Autodesk Inventor part; units mm, degrees
ref_plane "YZ Plane" through (0, 0, 0) normal (1, 0, 0) x (0, 1, 0)
ref_plane "XZ Plane" through (0, 0, 0) normal (0, 1, 0) x (-1, 0, 0)
ref_plane "XY Plane" through (0, 0, 0) normal (0, 0, 1) x (1, 0, 0)
sketch "Skizze1" plane through (0, 0, 0) normal (0, 1, 0) x (-1, 0, 0)
  line L0 (0, 0) -> (20, 0)
  line L1 (20, 0) -> (20, 40)
  line L2 (20, 40) -> (0, 40)
  line L3 (0, 40) -> (0, 0)
  circle A0 centre (10, 33) radius 2.55
  circle A1 centre (10, 7) radius 2.55
  dimension "d0" = 20
  dimension "d1" = 40
  dimension "d2" = 5.1
  dimension "d3" = 5.1
  dimension "d4" = 7
  dimension "d5" = 7
  dimension "d6" = 10
  dimension "d7" = 10
extrude "Extrusion1" add sketch "Skizze1" along normal blind 5
fillet "Rundung1" radius 2 4 edges at (-20, 2.5, 40) (-20, 2.5, 0) (0, 2.5, 0) (0, 2.5, 40)
sketch "Skizze2" plane through (0, 5, 0) normal (0, 1, 0) x (1, 0, 0)
  line L0 (-20, -2) -> (-20, -38)
  line L1 (-20, -25) -> (0, -25)
  line L2 (0, -25) -> (0, -15)
  line L3 (0, -15) -> (-20, -15)
  line L4 (-20, -15) -> (-20, -25)
  line L5 (-2, 0) -> (-18, 0)
  line L6 (-18, -40) -> (-2, -40)
  point P0 (0, 0)
  dimension "d11" = 10
  dimension "d12" = 20
  dimension "d13" = 15
  dimension "d14" = 15
sketch "Skizze5" plane through (0, 0, 0) normal (1, 0, 0) x (0, 1, 0)
  line L0 (55, 21) -> (55, 19)
  line L1 (5, 0) -> (0, 0)
  line L2 (5, 2) -> (5, 38)
  line L3 (5, 25) -> (55, 21)
  line L4 (5, 15) -> (55, 19)
  point P0 (5, 15)
  dimension "d25" = 19
  dimension "d26" = 2
  dimension "d27" = 50
extrude "Extrusion3" add sketch "Skizze5" against normal up to surface (20 mm away)
sketch "Skizze6" plane through (0, 55, 21) normal (0, 1, 0) x (1, 0, 0)
  line L0 (-20, 2) -> (0, 2)
  line L1 (0, 2) -> (0, 0)
  line L2 (0, 0) -> (-20, 0)
  line L3 (-20, 0) -> (-20, 2)
  point P0 (0, 21)
extrude "Extrusion4" add sketch "Skizze6" along normal blind 5
fillet "Rundung2" radius 2 2 edges at (-10, 5, 15) (-10, 5, 25)
fillet "Rundung3" radius 0.5 2 edges at (-10, 60, 21) (-10, 60, 19)
equation "\"d3\" = d2"
equation "\"d5\" = d4"
equation "\"d6\" = d7"
properties part number "Endtstop_Z" material "Polyaryletherketon-Kunststoff"
Model file for the job. Use its own axes, mm. A direction names the side the tool comes from. Give positions to 0.01 mm unless a question says otherwise; leave off trailing zeros. Loops run counter-clockwise (first coordinate to the right, second up) from the corner with the lowest first, then second, coordinate; pieces in that order, holes last. Notation, with made-up numbers: M 78,-24.5 L 128,-24.5 A25 cw 128,12.5 Z; hole C 21,75 d7. An arc over 180 degrees is marked long. Use one line per item in the form item = value.
Item 1: Slice it at C-C on x = -6.75. List the corners of the cut face in (y, z).
Filled in:
outline = M 0,0 L 5,0 L 5,13.15 A2 cw 6.84,15.15 L 55,19 L 59.5,19 A0.5 ccw 60,19.5 L 60,20.5 A0.5 ccw 59.5,21 L 55,21 L 6.84,24.85 A2 cw 5,26.85 L 5,40 L 0,40 Z
Item 2: Slice it at D-D on y = 44. List the corners of the cut face in (x, z).
Filled in:
outline = M -20,18.12 L 0,18.12 L 0,21.88 L -20,21.88 Z
Item 3: Which spindle directions (+Z, -Z, +X, -X, +Y, -Y) get a long thin tool onto all of the face, cutting with end or side? Do faces 1 (the flat face through (-8, 5, 5)), 2 (the flat face through (-10, 57, 21)), 3 (the cylindrical face through (-19.4, 2.54, 0.57)). Say none if no direction does.
Filled in:
face_1 = -Z, +X, -X, +Y
face_2 = +Z, +X, -X, +Y
face_3 = -Z, -X, +Y, -Y
Item 4: Slice it at A-A on z = 7. List the corners of the cut face in (x, y), and give its area (3 significant figures).
Filled in:
outline = M -20,0 L -12.55,0 L -12.55,5 L -20,5 Z; M -7.45,0 L 0,0 L 0,5 L -7.45,5 Z
area = 74.5 mm^2
Item 5: Drill centre lines: L1, parallel to Z at x = -10, y = 3.9; L2, parallel to Y at x = -1.25, z = 11; L3, parallel to Z at x = -13.5, y = 18.5. Where is each one in solid material? Low to high.
Filled in:
L1 = 0 to 4.45, 9.55 to 30.45, 35.55 to 40
L2 = 0 to 5
L3 = 16.08 to 23.92
Item 6: Flat gauge pins, fed straight in: pin 1 Ø4 at (x, z) = (-13, 34) entering from +Y; pin 2 Ø2 at (x, y) = (-8.5, 8) entering from -Z; pin 3 Ø5 at (x, z) = (-6.5, 10) entering from -Y; pin 4 Ø3 at (x, z) = (-10, 7) entering from +Y. Where does each tip first touch, or does it go through?
Filled in:
pin_1 = 5
pin_2 = 15.16
pin_3 = 0
pin_4 = through
Item 7: Slice it at B-B on x = -10. List the corners of the cut face in (y, z).
Filled in:
outline = M 0,0 L 5,0 L 5,4.45 L 0,4.45 Z; M 0,9.55 L 5,9.55 L 5,13.15 A2 cw 6.84,15.15 L 55,19 L 59.5,19 A0.5 ccw 60,19.5 L 60,20.5 A0.5 ccw 59.5,21 L 55,21 L 6.84,24.85 A2 cw 5,26.85 L 5,30.45 L 0,30.45 Z; M 0,35.55 L 5,35.55 L 5,40 L 0,40 Z
Item 8: Two-plate mould, pull along X, no slides. Class faces 4 (the cylindrical face through (-9.67, 2.46, 30.47)), 5 (the cylindrical face through (-11.18, 2.46, 9.26)), 6 (the flat face through (-20, 17, 21)), 7 (the flat face through (-10, 0, 20)): released by +X, released by -X, zero draft, split by the parting line, or undercut.
Filled in:
face_4 = undercut
face_5 = undercut
face_6 = released by -X
face_7 = zero draft
